Geometry: final body of the model. Coordinates: model frame, mm. Face numbers are marked on the shaded views. A direction names the side the tool comes from. Coordinates: 2 decimals unless noted, no trailing zeros. Write each loop counter-clockwise with the first axis right and the second up, starting at its lowest first coordinate (ties: lowest second). Pieces come first, ordered by that corner, then holes. Notation, with made-up numbers: (5, -26) -> (42, -26) arc R21 cw to (42, -10) -> close; hole circle Ø9 at (15, -14). An arc over 180 degrees is marked (long way). One line per item, written item: value.
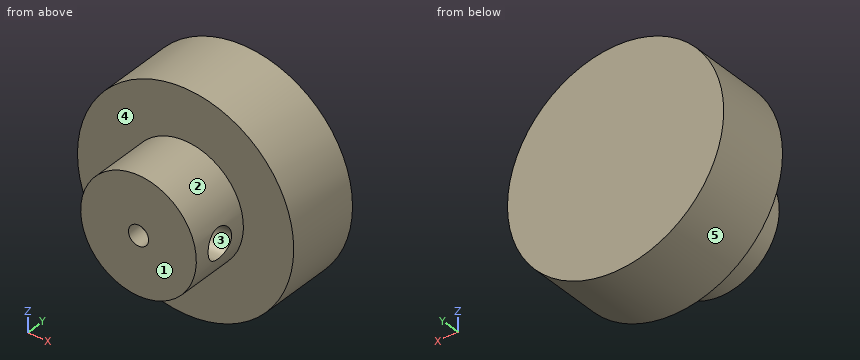
```python
from build123d import *

# Parameters (mm, degrees)
SKETCH4_R               = 3
CUT_EXTRUDE2_DEPTH      = 15
CUT_EXTRUDE2_DEPTH_BACK = 13


with BuildPart() as part:
    # Sketch1 → Revolve1 (revolve)
    with BuildSketch(Plane(origin=(0, 0, 0), x_dir=(0, 0, -1), z_dir=(1, 0, 0))):
        Polygon((2, 0), (21.5, 0), (21.5, -15), (11.5, -15), (11.5, -27), (2, -27), (2, -15), (0, -15), (0, 0), align=None)
    revolve(axis=Axis((0, 0, 0), (0, 1, 0)))

    # Sketch4 → Cut-Extrude2 (cut, two sides)
    with BuildSketch(Plane(origin=(0, 0, 0), x_dir=(0, 0, -1), z_dir=(1, 0, 0))) as cut_extrude2_sk:
        with Locations((0, -21)):
            Circle(SKETCH4_R)
    extrude(amount=CUT_EXTRUDE2_DEPTH, mode=Mode.SUBTRACT)
    extrude(cut_extrude2_sk.sketch, amount=-CUT_EXTRUDE2_DEPTH_BACK, mode=Mode.SUBTRACT)


solid = part.part
```
(1) First-contact query: pin 1 (7 mm diameter, centred on y = -21, z = 0, fed in from -X); pin 2 (4.5 mm diameter, centred on x = 0, z = -0.5, fed in from -Y); pin 3 (8 mm diameter, centred on y = -22, z = 14, fed in from -X); pin 4 (4 mm diameter, centred on x = -11, y = -14, fed in from +Z). Flat tips, straight axial feed; report the tip coordinate or a pass-through.
Responses:
pin 1: stops at x = -11.5
pin 2: stops at y = -27
pin 3: stops at x = -5.68
pin 4: stops at z = 19.53
(2) Section A-A (z = 0). Return the cut outline in (x, y).
Responses:
outline: (-21.5, -15) -> (-11.5, -15) -> (-11.5, -18) -> (-2, -18) -> (-2, -15) -> (2, -15) -> (2, -18) -> (11.5, -18) -> (11.5, -15) -> (21.5, -15) -> (21.5, 0) -> (-21.5, 0) -> close; (-11.5, -27) -> (-2, -27) -> (-2, -24) -> (-11.5, -24) -> close; (2, -27) -> (11.5, -27) -> (11.5, -24) -> (2, -24) -> close
(3) Pull-direction query (Z, two-part tool) for the marked faces 1, 2 and 3; classes: released by +Z, released by -Z, zero draft, split by the parting line, or undercut.
Responses:
face 1: zero draft
face 2: split by the parting line
face 3: undercut
(4) Section B-B (x = -8.5). Return the cut outline in (y, z), then the cut area to 3 significant figures.
Responses:
outline: (-27, -7.75) -> (-15, -7.75) -> (-15, -19.75) -> (0, -19.75) -> (0, 19.75) -> (-15, 19.75) -> (-15, 7.75) -> (-27, 7.75) -> close; hole circle Ø6 at (-21, 0)
area: 750 mm2
(5) Section D-D (y = -21). Return the cut outline in (x, z).
Responses:
outline: (-11.1, -3) arc R11.5 ccw to (11.1, -3) -> close; (-11.1, 3) -> (11.1, 3) arc R11.5 ccw to start
(6) Section C-C (x = 0). Return the cut outline in (y, z), then the cut area to 3 significant figures.
Responses:
outline: (-27, -11.5) -> (-15, -11.5) -> (-15, -21.5) -> (0, -21.5) -> (0, 21.5) -> (-15, 21.5) -> (-15, 11.5) -> (-27, 11.5) -> (-27, 2) -> (-23.24, 2) arc R3 cw to (-18.76, 2) -> (-15, 2) -> (-15, -2) -> (-18.76, -2) arc R3 cw to (-23.24, -2) -> (-27, -2) -> close
area: 867 mm2
(7) Line query: line 1 (Z direction, x = 0, y = -17.6); line 2 (Y direction, x = 3, z = 0). Output: solid intervals per line, ascending. Write a range as [from, to].
Responses:
line 1: z = [-11.5, -2], [2, 11.5]
line 2: y = [-27, -24], [-18, 0]
(8) Reachability of the marked faces 4 and 5 from +Z, -Z, +X, -X, +Y, -Y: full face, straight path, thin tool, end or side. Return the list, or none.
Responses:
face 4: -Y
face 5: +Y, -Y
